The model under review builds one solid part; all positions refer to its coordinate system, in mm. A direction names the side the tool comes from. Give positions to 0.01 mm unless a question says otherwise; leave off trailing zeros. Order: outer loops, then holes, each group sorted by start corner. A loop starts at its lowest first (then second) coordinate and runs counter-clockwise, first axis right, second up.
```python
from build123d import *

# Parameters (mm, degrees)
F1_DEPTH = 3


with BuildPart() as f1:
    # F0 (on Top) → F1 (new body)
    with BuildSketch(Plane.XY):
        Polygon((-112.926836, 0.004443), (-118.767626, 15.196789), (-124.284977, 0.394141), (-141.779017, 0.394141), (-127.85107, -9.025726), (-134.444977, -24.164799), (-130.936858, -22.362645), (-132.35915, -26.250625), (-152.67915, -26.250625), (-152.799174, -41.2316), (-137.323676, -41.2316), (-144.994139, -65.857825), (-138.929132, -66.758923), (-132.882882, -41.2316), (-130.191522, -40.962152), (-135.305133, -66.396103), (-129.567399, -67.605936), (-125.885266, -41.2316), (-123.300462, -40.97282), (-125.885266, -68.952925), (-120.098776, -72.956369), (-119.616715, -41.2316), (-116.962913, -40.965912), (-116.962913, -72.317163), (-110.744054, -68.574946), (-113.186582, -41.2316), (-110.90286, -41.2316), (-107.001505, -68.030101), (-101.292202, -66.602776), (-106.145109, -41.2316), (-104.622629, -41.2316), (-97.866622, -66.602776), (-91.776701, -65.36576), (-99.484258, -41.2316), (-84.670836, -40.97282), (-84.721535, -26.250625), (-102.501535, -26.250625), (-105.948821, -22.362645), (-102.935558, -24.450401), (-109.310944, -8.844978), (-95.608622, 0.004443), align=None)
        Polygon((-129.142605, -26.250625), (-127.429816, -20.12761), (-125.686861, -19.232238), (-127.287082, -26.250625), align=None, mode=Mode.SUBTRACT)
        Polygon((-123.898953, -26.163155), (-122.719641, -17.130227), (-121.70087, -16.606875), (-122.196288, -26.250625), align=None, mode=Mode.SUBTRACT)
        Polygon((-119.130578, -26.424788), (-118.767626, -14.656196), (-117.951181, -14.960507), (-117.390959, -26.250625), align=None, mode=Mode.SUBTRACT)
        Polygon((-114.525939, -26.416255), (-115.012083, -16.606875), (-113.727491, -17.701157), (-112.871551, -26.250625), align=None, mode=Mode.SUBTRACT)
        Polygon((-110.167341, -26.250625), (-110.833426, -19.597496), (-108.827006, -21.079161), (-107.999686, -26.250625), align=None, mode=Mode.SUBTRACT)
    extrude(amount=F1_DEPTH)


solid = f1.part
```
Item 1: Take a section at A-A (y = -60.5). Give the boundary of the cut face in (x, z).
Values found:
outline: (-143.33, 0) - (-137.45, 0) - (-137.45, 3) - (-143.33, 3) - close; (-134.12, 0) - (-128.58, 0) - (-128.58, 3) - (-134.12, 3) - close; (-125.1, 0) - (-119.91, 0) - (-119.91, 3) - (-125.1, 3) - close; (-116.96, 0) - (-111.47, 0) - (-111.47, 3) - (-116.96, 3) - close; (-108.1, 0) - (-102.46, 0) - (-102.46, 3) - (-108.1, 3) - close; (-99.49, 0) - (-93.33, 0) - (-93.33, 3) - (-99.49, 3) - close
Item 2: Clearance check with flat-ended pins moving along their axes: pin 1 Ø0.9 at (x, z) = (-144, 1) entering from -Y; pin 2 Ø1.5 at (x, z) = (-105.5, 1) entering from +Y; pin 3 Ø0.9 at (x, z) = (-89, 1) entering from +Y; pin 4 Ø5 at (x, y) = (-129.5, 3) entering from -Z. State where each tip first meets the part, or that it passes through.
Values found:
pin 1: stops at y = -66.07
pin 2: stops at y = 0
pin 3: stops at y = -26.25
pin 4: passes through
Item 3: Take a section at C-C (y = -47). Give the boundary of the cut face in (x, z), and give its area (3 significant figures).
Values found:
outline: (-139.12, 0) - (-134.25, 0) - (-134.25, 3) - (-139.12, 3) - close; (-131.41, 0) - (-126.69, 0) - (-126.69, 3) - (-131.41, 3) - close; (-123.86, 0) - (-119.7, 0) - (-119.7, 3) - (-123.86, 3) - close; (-116.96, 0) - (-112.67, 0) - (-112.67, 3) - (-116.96, 3) - close; (-110.06, 0) - (-105.04, 0) - (-105.04, 3) - (-110.06, 3) - close; (-103.09, 0) - (-97.64, 0) - (-97.64, 3) - (-103.09, 3) - close
area: 85.5 mm2
Item 4: Take a section at B-B (x = -140.5). Give the boundary of the cut face in (y, z).
Values found:
outline: (-66.53, 0) - (-51.43, 0) - (-51.43, 3) - (-66.53, 3) - close; (-41.23, 0) - (-26.25, 0) - (-26.25, 3) - (-41.23, 3) - close; (-0.47, 0) - (0.39, 0) - (0.39, 3) - (-0.47, 3) - close
Item 5: For line 1 (X direction, y = -60, z = 2.7); line 2 (X direction, y = -47, z = 2.95); line 3 (X direction, y = -29, z = 0.9), list the stretches that pass through material, from the lowest coordinate up.
Values found:
line 1: x = -143.17 to -137.33, -134.02 to -128.51, -125.06 to -119.9, -116.96 to -111.51, -108.17 to -102.56, -99.62 to -93.49
line 2: x = -139.12 to -134.25, -131.41 to -126.69, -123.86 to -119.7, -116.96 to -112.67, -110.06 to -105.04, -103.09 to -97.64
line 3: x = -152.7 to -84.71
Item 6: Draft analysis for pull direction Y (two halves, no side actions). For faces 4 (the flat face through (-119, -28, 0)), 5 (the flat face through (-123.036, -26.208, 1.479)), 6 (the flat face through (-94.9, -66, 1.5)), state which applies: released by +Y, released by -Y, zero draft, split by the parting line, or undercut.
Values found:
face 4: zero draft
face 5: undercut
face 6: released by -Y
Item 7: For faces 1 (the flat face through (-110.496, -22.971, 1.479)), 2 (the flat face through (-131.1, -16.49, 1.48)), 3 (the flat face through (-119, -28, 3)), list the 3-axis set-ups (+Z, -Z, +X, -X, +Y, -Y) from which the entire face can be reached by the end or side of a thin tool; tool diameter is ignored.
Values found:
face 1: +Z, -Z
face 2: +Z, -Z, -X
face 3: +Z, +X, -X, +Y, -Y
Item 8: Take a section at D-D (z = 1.95). Give the number of separate pieces and of enclosed holes in the cut face, and give its area (3 significant figures).
Values found:
separate pieces: 1
enclosed holes: 5
area: 2,610 mm2
